Part model, mm, in its own coordinate system. A direction names the side the tool comes from. Give positions to 0.01 mm unless a question says otherwise; leave off trailing zeros. Order: outer loops, then holes, each group sorted by start corner. A loop starts at its lowest first (then second) coordinate and runs counter-clockwise, first axis right, second up. Notation, with made-up numbers: M 84,0 L 111,0 A19 ccw 111,7 Z; hole C 20.5,8 d6. An arc over 180 degrees is marked long. Answer as a JSON object with one key per item and string values.
from build123d import *

# Parameters (mm, degrees)
SKETCH_1_W           = 29.3
SKETCH_1_H           = 29
EXTRUDE_1_DEPTH      = 2
SKETCH_2_R           = 1.75
CUT_EXTRUDE_1_DEPTH  = 2
SKETCH_3_R           = 1.1
CUT_EXTRUDE_2_DEPTH  = 2
SKETCH_4_W           = 29.3
SKETCH_4_H           = 2
EXTRUDE_2_DEPTH      = 30
EXTRUDE_2_DEPTH_BACK = 2
SKETCH_5_R           = 3.25
CUT_EXTRUDE_3_DEPTH  = 30


with BuildPart() as part:
    # 草图1 → 凸台-拉伸1 (new body)
    with BuildSketch(Plane.XY):
        Rectangle(SKETCH_1_W, SKETCH_1_H)
    extrude(amount=EXTRUDE_1_DEPTH)

    # 草图2 → 切除-拉伸1 (cut)
    with BuildSketch(Plane.XY.offset(2)):
        with Locations((-11.65, 10)):
            Circle(SKETCH_2_R)
        with Locations((-11.65, -10)):
            Circle(SKETCH_2_R)
        with Locations((12.05, 0)):
            Circle(SKETCH_2_R)
    extrude(amount=-CUT_EXTRUDE_1_DEPTH, mode=Mode.SUBTRACT)

    # 草图3 → 切除-拉伸2 (cut)
    with BuildSketch(Plane.XY.offset(2)):
        with Locations((-10.15, 5.995187484)):
            Circle(SKETCH_3_R)
        with Locations((-10.15, -6.004812516)):
            Circle(SKETCH_3_R)
        with Locations((11.85, 5.995187484)):
            Circle(SKETCH_3_R)
        with Locations((11.85, -6.004812516)):
            Circle(SKETCH_3_R)
    extrude(amount=-CUT_EXTRUDE_2_DEPTH, mode=Mode.SUBTRACT)

    # 草图4 → 凸台-拉伸2 (add, two sides)
    with BuildSketch(Plane.XY.offset(2)) as extrude_2_sk:
        with Locations((0, 15.5)):
            Rectangle(SKETCH_4_W, SKETCH_4_H)
    extrude(amount=EXTRUDE_2_DEPTH)
    extrude(extrude_2_sk.sketch, amount=-EXTRUDE_2_DEPTH_BACK)

    # 草图5 → 切除-拉伸3 (cut)
    with BuildSketch(Plane.XZ.offset(-14.5)):
        with Locations((0.35, 17)):
            Circle(SKETCH_5_R)
    extrude(amount=-CUT_EXTRUDE_3_DEPTH, mode=Mode.SUBTRACT)


solid = part.part
1. Cut at D-D on y = -6.5. Give the cut face in (x, z), plus the area to 3 significant figures.
Worked answers:
{"outline": "M -14.65,0 L -11.13,0 L -11.13,2 L -14.65,2 Z; M -9.17,0 L 10.87,0 L 10.87,2 L -9.17,2 Z; M 12.83,0 L 14.65,0 L 14.65,2 L 12.83,2 Z", "area": "50.7 mm^2"}
2. Cut at A-A on x = 0.35. Give the cut face in (y, z).
Worked answers:
{"outline": "M -14.5,0 L 16.5,0 L 16.5,13.75 L 14.5,13.75 L 14.5,2 L -14.5,2 Z; M 14.5,20.25 L 16.5,20.25 L 16.5,32 L 14.5,32 Z"}
3. Probe line 1 along Y through (x, z) = (-11.65, 0.75); line 2 along Y through (x, z) = (12.05, 0.55); line 3 along Y through (x, z) = (-8.5, 23.5). List the from-to ranges inside material, lowest first.
Worked answers:
{"line 1": "y = -14.5 to -11.75, -8.25 to 8.25, 11.75 to 16.5", "line 2": "y = -14.5 to -7.09, -4.92 to -1.75, 1.75 to 4.91, 7.08 to 16.5", "line 3": "y = 14.5 to 16.5"}
4. Pin check, flat tips, straight feed: P1, Ø5.5, axis at x = 12.05, y = 0, coming from the +Z side; P2, Ø9, axis at x = -5.5, z = 10, coming from the -Y side. Stop position of each tip, or through.
Worked answers:
{"P1": "stops at z = 2", "P2": "stops at y = 14.5"}
5. Cut at B-B on y = 0. Give the cut face in (x, z).
Worked answers:
{"outline": "M -14.65,0 L 10.3,0 L 10.3,2 L -14.65,2 Z; M 13.8,0 L 14.65,0 L 14.65,2 L 13.8,2 Z"}
6. Two-plate mould, pull along X, no slides. Class faces 1 (the cylindrical face through (-11, -6.7, 1)), 2 (the flat face through (0, -14.5, 1)), 3 (the flat face through (-14.65, 15, 9)), 4 (the flat face through (14.65, 15, 9)): +X half, -X half, draft (parallel to the pull), parting line (faces both ways), or undercut.
Worked answers:
{"face 1": "undercut", "face 2": "draft", "face 3": "-X half", "face 4": "+X half"}
7. Cut at C-C on z = 17. Give the cut face in (x, y), plus the area to 3 significant figures.
Worked answers:
{"outline": "M -14.65,14.5 L -2.9,14.5 L -2.9,16.5 L -14.65,16.5 Z; M 3.6,14.5 L 14.65,14.5 L 14.65,16.5 L 3.6,16.5 Z", "area": "45.6 mm^2"}
8. Which spindle directions (+Z, -Z, +X, -X, +Y, -Y) get a long thin tool onto all of the face, cutting with end or side? Do faces 5 (the cylindrical face through (-0.073, 15.486, 20.222)), 6 (the flat face through (0, 0, 2)). Say none if no direction does.
Worked answers:
{"face 5": "+Y, -Y", "face 6": "+Z, +X, -X, -Y"}
